```python
from build123d import *

# Parameters (mm, degrees)
BOSS_EXTRUDE1_DEPTH = 3.175
SKETCH5_R           = 1.5875
CUT_EXTRUDE1_DEPTH  = 4.175


with BuildPart() as part:
    # Sketch2 → Boss-Extrude1 (new body)
    with BuildSketch(Plane(origin=(0, 0, 0), x_dir=(1, 0, 0), z_dir=(0, 1, 0))):
        with BuildLine():
            Line((-64.433559451, -10.720044429), (-64.433559451, -74.220044429))
            ThreePointArc((-64.433559451, -74.220044429), (-60.115559451, -78.538044429), (-55.797559451, -74.220044429))
            Line((-55.797559451, -74.220044429), (-55.797559451, -10.720044429))
            ThreePointArc((-55.797559451, -10.720044429), (-35.103902349, 15.133874618), (-5.345262109, 0.605423034))
            ThreePointArc((-5.345262109, 0.605423034), (0.404037892, -1.452682281), (2.462143207, 4.296617721))
            ThreePointArc((2.462143207, 4.296617721), (-36.995428675, 23.560180104), (-64.433559451, -10.720044429))
        make_face()
    extrude(amount=BOSS_EXTRUDE1_DEPTH)

    # Sketch5 → Cut-Extrude1 (cut, through all)
    with BuildSketch(Plane(origin=(0, 3.175, 0), x_dir=(1, 0, 0), z_dir=(0, 1, 0))):
        with Locations((-26.841559451, 19.723020377)):
            Circle(SKETCH5_R)
        with Locations((-1.441559451, 2.451020377)):
            Circle(SKETCH5_R)
    extrude(amount=-CUT_EXTRUDE1_DEPTH, mode=Mode.SUBTRACT)


solid = part.part
```
The listing builds one solid part. Answer for the finished solid, in the listing's coordinates (mm). Round coordinates to 2 decimals unless told otherwise and drop trailing zeros. Loops run counter-clockwise (first coordinate to the right, second up) from the corner with the lowest first, then second, coordinate; pieces in that order, holes last. Notation, with made-up numbers: (-32.5, 38.25) -> (-25.5, 38.25) arc R13 ccw to (-25.5, 57.25) -> close; hole circle Ø1 at (75, 45). An arc over 180 degrees is marked (long way). Use one line per item in the form item = value.
1. Find the intervals of material crossed by probe 1 along X at (y, z) = (1.85, 32.5); probe 2 along X at (y, z) = (1.4, -13); probe 3 along Z at (x, y) = (-25.5, 1.6), in increasing order. Write a range as [from, to].
Answer key:
probe_1 = [-64.43, -55.8]
probe_2 = [-55.22, -41.11], [-17.49, -3.38]
probe_3 = [-24.21, -20.57], [-18.87, -15.5]
2. The part is cut by section C-C on z = 63.5. Determine the outline of the cut face in (x, y) (3 decimals).
Answer key:
outline = (-64.434, 0) -> (-55.798, 0) -> (-55.798, 3.175) -> (-64.434, 3.175) -> close
3. The part is cut by section A-A on x = -26.5. Determine the outline of the cut face in (y, z) (1 decimal), and give its area (3 significant figures).
Answer key:
outline = (0, -24.3) -> (3.2, -24.3) -> (3.2, -21.3) -> (0, -21.3) -> close; (0, -18.2) -> (3.2, -18.2) -> (3.2, -15.6) -> (0, -15.6) -> close
area = 17.7 mm²
4. The part is cut by section B-B on y = 2.4. Determine the outline of the cut face in (x, z) (1 decimal).
Answer key:
outline = (-64.4, 10.7) arc R35.1 ccw to (2.5, -4.3) arc R4.3 ccw to (-5.3, -0.6) arc R26.5 cw to (-55.8, 10.7) -> (-55.8, 74.2) arc R4.3 ccw to (-64.4, 74.2) -> close; hole circle Ø3.2 at (-26.8, -19.7); hole circle Ø3.2 at (-1.4, -2.5)
5. The part is cut by section D-D on x = -46.5. Determine the outline of the cut face in (y, z) (3 decimals).
Answer key:
outline = (0, -19.915) -> (3.175, -19.915) -> (3.175, -9.436) -> (0, -9.436) -> close
6. For a pull along Z with two mould halves and no side action, classify faces 1 (the cylindrical face through (-27.186, 1.61, -18.173)), 2 (the flat face through (-55.798, 2, 43)), 3 (the cylindrical face through (-60.211, 1.565, 78.537)) as released by +Z, released by -Z, zero draft, split by the parting line, or undercut.
Answer key:
face_1 = undercut
face_2 = zero draft
face_3 = released by +Z
7. A flat-ended cylindrical pin translates along its axis: pin 1 Ø1 at (y, z) = (1.5, 27) entering from +X. Find the tip coordinate at first contact, or state that the pin passes through.
Answer key:
pin_1 = -55.8
